from build123d import *

# Parameters (mm, degrees)
SKETCH1_R                = 12.4187
BOSS_EXTRUDE1_DEPTH      = 80
SKETCH1_3_R              = 9.9187
CUT_EXTRUDE1_DEPTH       = 20
BOSS_EXTRUDE2_REACH      = 86.682
BOSS_EXTRUDE2_END_RADIUS = 12.4187
SKETCH2_W                = 24
SKETCH2_H                = 4.51281607
SKETCH3_R                = 0.6
CUT_EXTRUDE2_DEPTH       = 10


with BuildPart() as part:
    # Sketch1 → Boss-Extrude1 (new body)
    with BuildSketch(Plane(origin=(0, 0, 0), x_dir=(1, 0, 0), z_dir=(0, 1, 0))):
        with Locations(Location((0, 0, 0), (0, 0, 270))):
            Circle(SKETCH1_R)
    extrude(amount=-BOSS_EXTRUDE1_DEPTH)

    # Sketch1_3 → Cut-Extrude1 (cut)
    with BuildSketch(Plane(origin=(0, 0, 0), x_dir=(1, 0, 0), z_dir=(0, 1, 0))):
        with Locations(Location((0, 0, 0), (0, 0, 270))):
            Circle(SKETCH1_3_R)
    extrude(amount=-CUT_EXTRUDE1_DEPTH, mode=Mode.SUBTRACT)

    # Boss-Extrude2: up to this cylinder (the profile starts outside it)
    boss_extrude2_end = Plane(origin=(0, -76.743592, 0), z_dir=(0, 1, 0)) * Cylinder(BOSS_EXTRUDE2_END_RADIUS, 199.2014, mode=Mode.PRIVATE)
    # Sketch2 → Boss-Extrude2 (add, up to the surface)
    with BuildSketch(Plane.XY.offset(-12.4187), mode=Mode.PRIVATE) as boss_extrude2_sk1:
        with Locations((0, -76.743591965)):
            Rectangle(SKETCH2_W, SKETCH2_H)
    boss_extrude2_tool1 = extrude(boss_extrude2_sk1.sketch, amount=BOSS_EXTRUDE2_REACH, mode=Mode.PRIVATE) - boss_extrude2_end
    add(boss_extrude2_tool1.solids().sort_by_distance((0, -76.743592, -12.4187))[0])
    add(boss_extrude2_tool1.solids().sort_by_distance((0, -76.743592, -12.4187))[1])

    # Sketch3 → Cut-Extrude2 (cut)
    with BuildSketch(Plane(origin=(0, 0, -12.4187), x_dir=(-1, 0, 0), z_dir=(0, 0, -1))):
        with Locations((-4.45, -76.743591965)):
            Circle(SKETCH3_R)
        with Locations((-6.45, -76.743591965)):
            Circle(SKETCH3_R)
        with Locations((-8.45, -76.743591965)):
            Circle(SKETCH3_R)
        with Locations((-10.45, -76.743591965)):
            Circle(SKETCH3_R)
        with Locations(Location((10.45, -76.743591965, 0), (0, 0, 180))):
            Circle(SKETCH3_R)
        with Locations(Location((8.45, -76.743591965, 0), (0, 0, 180))):
            Circle(SKETCH3_R)
        with Locations(Location((6.45, -76.743591965, 0), (0, 0, 180))):
            Circle(SKETCH3_R)
        with Locations(Location((4.45, -76.743591965, 0), (0, 0, 180))):
            Circle(SKETCH3_R)
    extrude(amount=-CUT_EXTRUDE2_DEPTH, mode=Mode.SUBTRACT)


solid = part.part
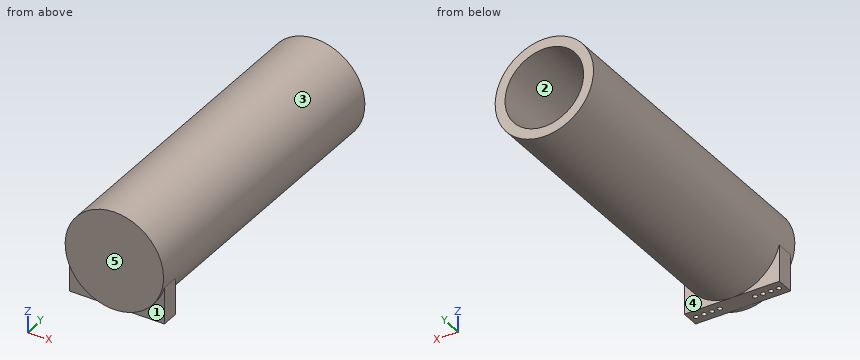
Can you work these out from the model? Positions are in its coordinate system, mm. Face numbers are marked on the shaded views. A direction names the side the tool comes from. Give positions to 0.01 mm unless a question says otherwise; leave off trailing zeros. Loops run counter-clockwise (first coordinate to the right, second up) from the corner with the lowest first, then second, coordinate; pieces in that order, holes last. Notation, with made-up numbers: (22.25, -3.75) - (59.25, -3.75) arc R17 cw to (59.25, 12.25) - close; hole circle Ø11 at (19, 32). An arc over 180 degrees is marked (long way). One line per item, written item: value.
(1) If we section it at B-B, the plane y = -7: List the corners of the cut face in (x, z) for me.
Verdict:
outline: circle Ø24.84 at (0, 0); hole circle Ø19.84 at (0, 0)
(2) If we mould it in two halves opening along X, with no side actions, what happens to the marked faces 1, 2 and 3? For each: released by +X, released by -X, zero draft, split by the parting line, or undercut.
Verdict:
face 1: zero draft
face 2: undercut
face 3: split by the parting line
(3) If we section it at D-D, the plane y = -38.5: List the corners of the cut face in (x, z) for me, plus the area to 3 significant figures.
Verdict:
outline: circle Ø24.84 at (0, 0)
area: 485 mm^2
(4) If we section it at C-C, the plane z = -8.5: State how many separate pieces and enclosed holes the cut face has, plus the area to 3 significant figures.
Verdict:
separate pieces: 1
enclosed holes: 8
area: 1,260 mm^2
(5) I need wall thicknesses on line 1 along Y through (x, z) = (4.45, -8.25); line 2 along Y through (x, z) = (-10.45, -8.5); line 3 along Y through (x, z) = (0.5, 0.75). Which ranges of each line are inside material? Lowest first, please.
Verdict:
line 1: -80 to -77.34, -76.14 to -20
line 2: -79 to -77.34, -76.14 to -74.49
line 3: -80 to -20
(6) On a 3-axis mill with a long thin cutter (end or side, diameter ignored), from which of +Z, -Z, +X, -X, +Y, -Y can I reach the whole of each face in a straight line? I mean the marked faces 4 and 5. Say none if no direction works.
Verdict:
face 4: -Z, +X, +Y
face 5: +Z, -Z, +X, -X, -Y
(7) If we section it at A-A, the plane z = 0: List the corners of the cut face in (x, y) for me.
Verdict:
outline: (-12.42, -80) - (12.42, -80) - (12.42, 0) - (9.92, 0) - (9.92, -20) - (-9.92, -20) - (-9.92, 0) - (-12.42, 0) - close
(8) I'm going to push flat-ended pins straight in: pin 1 (1.5 mm diameter, centred on x = -9.5, y = -46.5, fed in from -Z); pin 2 (6 mm diameter, centred on x = 8.5, y = -54.5, fed in from +Z); pin 3 (4 mm diameter, centred on y = -64, z = -2.5, fed in from +X). Where does each tip first touch, or does it pass through?
Verdict:
pin 1: z = -8.81
pin 2: z = 11.13
pin 3: x = 12.41
